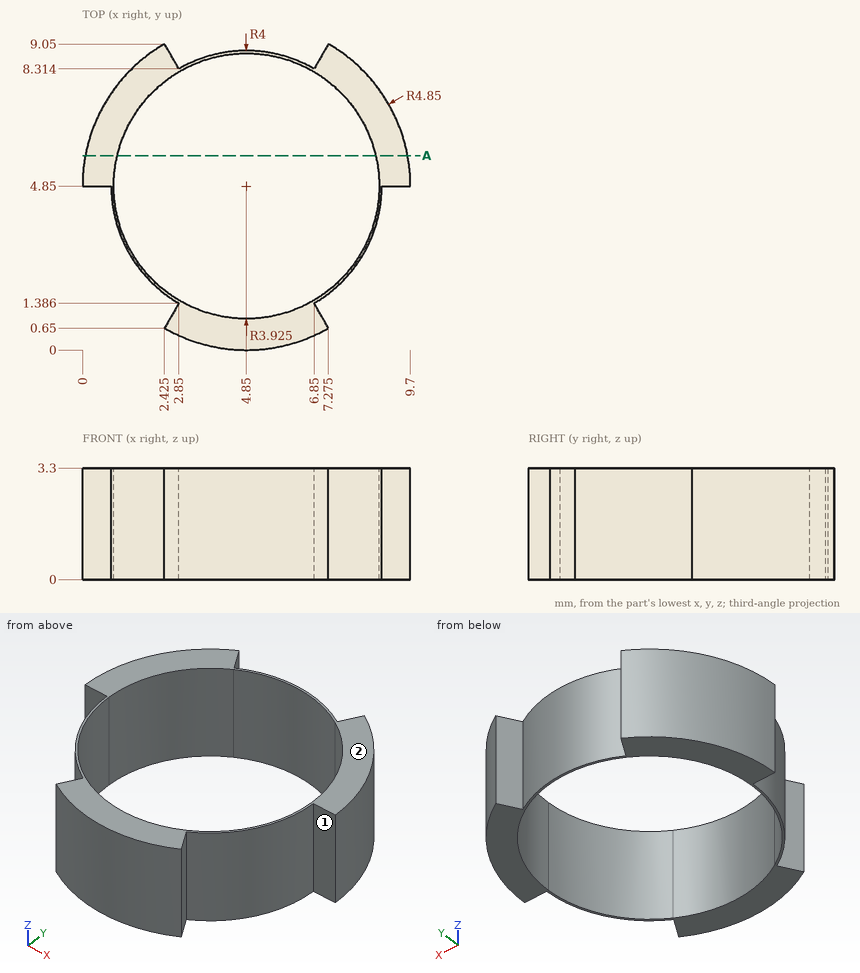
Input: dimensioned drawing with shaded views. Units: mm. Origin: part minimum x, y, z. A direction names the side the tool comes from. Coordinates: 2 decimals unless noted, no trailing zeros. Loops run counter-clockwise (first coordinate to the right, second up) from the corner with the lowest first, then second, coordinate; pieces in that order, holes last. Notation, with made-up numbers: (-4, 66.25) -> (49, 66.25) arc R14 ccw to (49, 93.25) -> close; hole circle Ø10 at (5, 57). An arc over 180 degrees is marked (long way). Use a Markdown table: item, result. Add a question column.
(1) Section query A-A, the plane y = 5.75. Return loops of the section in (x, z).
(2) Line query: line 1 along X through (y, z) = (5, 3.1); line 2 along X through (y, z) = (5.75, 3.05); line 3 along Y through (x, z) = (0.75, 0.7). Output: solid intervals per line, ascending.
(3) Access query for the marked faces 1 and 2. Directions: +Z, -Z, +X, -X, +Y, -Y. A direction counts if a zero-diameter tool reaches every point of the face in a straight line with its end or side. Return the directions, or none.
(4) Pin query (flat end, axial travel): pin 1 Ø0.7 at (x, z) = (9.5, 1.5) entering from -Y. Return the tip coordinate at first contact, or that it passes through.
Answer:
| question | item | result |
|---|---|---|
| 1 | outline | (0.08, 0) -> (1.03, 0) -> (1.03, 3.3) -> (0.08, 3.3) -> close; (8.67, 0) -> (9.62, 0) -> (9.62, 3.3) -> (8.67, 3.3) -> close |
| 2 | line 1 | x = 0 to 0.93, 8.77 to 9.7 |
| 2 | line 2 | x = 0.08 to 1.03, 8.67 to 9.62 |
| 2 | line 3 | y = 4.85 to 7.44 |
| 3 | face 1 | +Z, -Z, +X, -Y |
| 3 | face 2 | +Z, +X, -X, +Y, -Y |
| 4 | pin 1 | stops at y = 4.85 |
